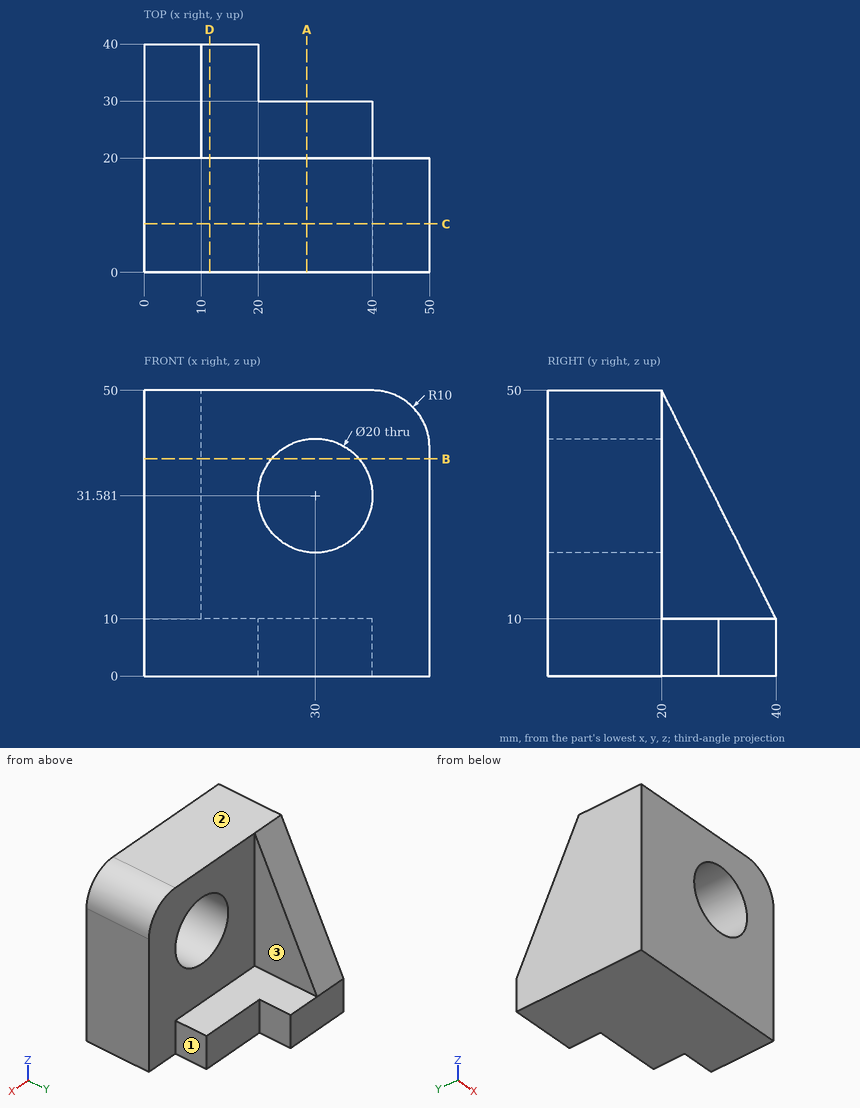
Here's the drawing with two shaded views (mm, measured from the low corner). I have some questions. A direction names the side the tool comes from. Coordinates: 2 decimals unless noted, no trailing zeros. Order: outer loops, then holes, each group sorted by start corner. A loop starts at its lowest first (then second) coordinate and runs counter-clockwise, first axis right, second up. Notation, with made-up numbers: (9, -12.75) - (14, -12.75) arc R24 ccw to (14, -0.75) - close; hole circle Ø9 at (-18.75, 19.5). An arc over 180 degrees is marked (long way). Answer in a Markdown table with one row per item.
1. Suppose I cut it at D-D (x = 11.5). Please give me the cut outline in (y, z).
Reply:
| item | result |
|---|---|
| outline | (0, 0) - (40, 0) - (40, 10) - (20, 10) - (20, 50) - (0, 50) - close |
2. Suppose I cut it at B-B (z = 38). Please give me the cut outline in (x, y).
Reply:
| item | result |
|---|---|
| outline | (0, 0) - (22.33, 0) - (22.33, 20) - (10, 20) - (10, 26) - (0, 26) - close; (37.67, 0) - (50, 0) - (50, 20) - (37.67, 20) - close |
3. For the marked faces 1, 2 and 3, which set-ups out of +Z, -Z, +X, -X, +Y, -Y let a thin tool reach every point of the face, with its end or its side?
Reply:
| item | result |
|---|---|
| face 1 | +Z, -Z, +X, +Y |
| face 2 | +Z, +X, -X, +Y, -Y |
| face 3 | +Z, +X, +Y |
4. If I drill on line 1 along X through (y, z) = (28, 24.5); line 2 along Y through (x, z) = (20, 22.5); line 3 along Z through (x, y) = (27, 2.5), over which ranges is the centre line in solid material (lowest first)?
Reply:
| item | result |
|---|---|
| line 1 | x = 0 to 10 |
| line 2 | y = 0 to 20 |
| line 3 | z = 0 to 22.04, 41.12 to 50 |
5. Suppose I cut it at A-A (x = 28.5). Please give me the cut outline in (y, z).
Reply:
| item | result |
|---|---|
| outline | (0, 0) - (30, 0) - (30, 10) - (20, 10) - (20, 21.69) - (0, 21.69) - close; (0, 41.47) - (20, 41.47) - (20, 50) - (0, 50) - close |
6. Suppose I cut it at C-C (y = 8.5). Please give me the cut outline in (x, z), and give its area (3 significant figures).
Reply:
| item | result |
|---|---|
| outline | (0, 0) - (50, 0) - (50, 40) arc R10 ccw to (40, 50) - (0, 50) - close; hole circle Ø20 at (30, 31.58) |
| area | 2,160 mm^2 |
7. For pin 1 (11 mm diameter, centred on y = 33, z = 7.5, fed in from +X); pin 2 (12 mm diameter, centred on x = 33, z = 37.5, fed in from +Y); pin 3 (11 mm diameter, centred on x = 30, z = 4.5, fed in from +Y); pin 4 (2 mm diameter, centred on x = 10.5, y = 20.5, fed in from +Z), each with a flat end and sliding along its axis, tell me the tip position at first contact or that it passes through.
Reply:
| item | result |
|---|---|
| pin 1 | stops at x = 40 |
| pin 2 | stops at y = 20 |
| pin 3 | stops at y = 30 |
| pin 4 | stops at z = 50 |
